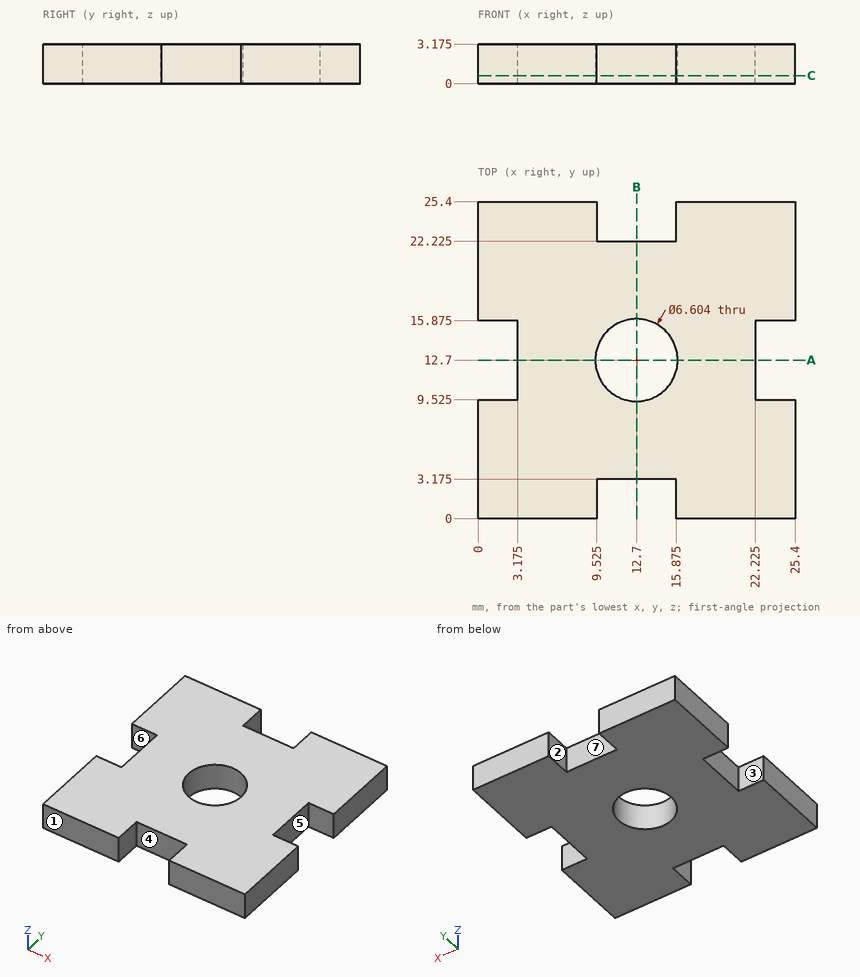
Geometry: see drawing. Coordinates: mm, zero at the bounding-box minimum. A direction names the side the tool comes from. Coordinates: 2 decimals unless noted, no trailing zeros. Loops run counter-clockwise (first coordinate to the right, second up) from the corner with the lowest first, then second, coordinate; pieces in that order, holes last. Notation, with made-up numbers: (-35.5, -28.5) - (-28.5, -28.5) arc R31 cw to (-28.5, 1.5) - close; hole circle Ø8 at (-30.5, -37.5). An arc over 180 degrees is marked (long way). Return JSON: item names as keys, results as strings.
Q1. Access query for the marked faces 4, 5, 6 and 7. Directions: +Z, -Z, +X, -X, +Y, -Y. A direction counts if a zero-diameter tool reaches every point of the face in a straight line with its end or side. Return the directions, or none.
Results:
{"face 4": "+Z, -Z, -Y", "face 5": "+Z, -Z, +X", "face 6": "+Z, -Z, -X", "face 7": "+Z, -Z, +Y"}
Q2. Mould query, pull axis Y, two halves, no side actions, for the marked faces 1, 2 and 3. Classes: released by +Y, released by -Y, zero draft, split by the parting line, or undercut.
Results:
{"face 1": "released by -Y", "face 2": "zero draft", "face 3": "undercut"}
Q3. Section A-A, the plane y = 12.7. Return loops of the section in (x, z) (3 decimals), plus the area to 3 significant figures.
Results:
{"outline": "(3.175, 0) - (9.398, 0) - (9.398, 3.175) - (3.175, 3.175) - close; (16.002, 0) - (22.225, 0) - (22.225, 3.175) - (16.002, 3.175) - close", "area": "39.5 mm2"}
Q4. Material intervals for line 1 along Y through (x, z) = (12.75, 0.4) (3 decimals); line 2 along X through (y, z) = (24, 2.7) (3 decimals), sorted ascending.
Results:
{"line 1": "3.175 to 9.398, 16.002 to 22.225", "line 2": "0 to 9.525, 15.875 to 25.4"}
Q5. Contact query for a flat-ended pin moving along its axis: P1, Ø1.6, axis at y = 11.5, z = 2, coming from the +X side (3 decimals). Output: stop coordinate, or through.
Results:
{"P1": "x = 22.225"}
Q6. Section C-C, the plane z = 0.65. Return loops of the section in (x, y) (3 decimals), plus the area to 3 significant figures.
Results:
{"outline": "(0, 0) - (9.525, 0) - (9.525, 3.175) - (15.875, 3.175) - (15.875, 0) - (25.4, 0) - (25.4, 9.525) - (22.225, 9.525) - (22.225, 15.875) - (25.4, 15.875) - (25.4, 25.4) - (15.875, 25.4) - (15.875, 22.225) - (9.525, 22.225) - (9.525, 25.4) - (0, 25.4) - (0, 15.875) - (3.175, 15.875) - (3.175, 9.525) - (0, 9.525) - close; hole circle Ø6.604 at (12.7, 12.7)", "area": "530 mm2"}
